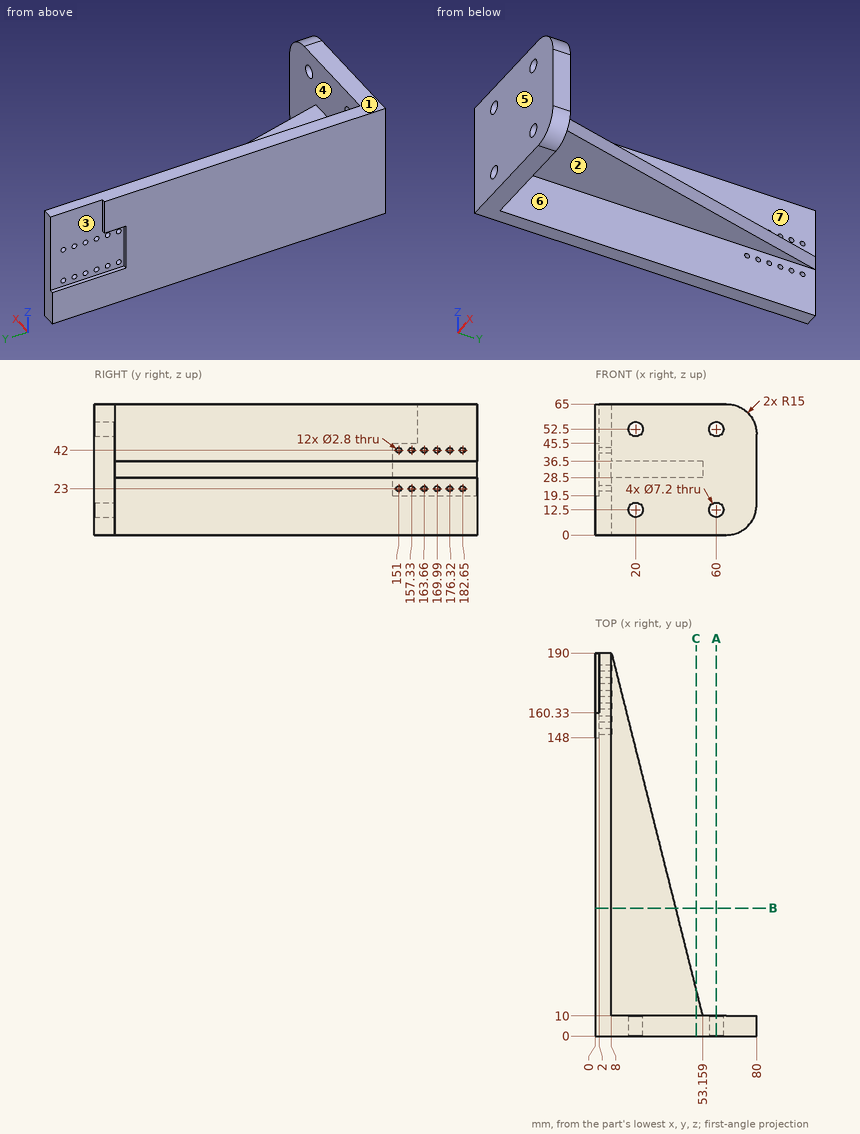
Can you work these out from the drawing? Everything is in mm from the part's minimum corner. A direction names the side the tool comes from. Round coordinates to 2 decimals unless told otherwise and drop trailing zeros. Loops run counter-clockwise (first coordinate to the right, second up) from the corner with the lowest first, then second, coordinate; pieces in that order, holes last. Notation, with made-up numbers: (3, 70) - (39, 70) arc R30 cw to (39, 98) - close; hole circle Ø10 at (85.25, -10.75). An arc over 180 degrees is marked (long way). Answer in a Markdown table with one row per item. Add a question column.
(1) I'm going to push flat-ended pins straight in: pin 1 (6.5 mm diameter, centred on x = 60, z = 52.5, fed in from -Y); pin 2 (12 mm diameter, centred on x = 64.5, z = 44.5, fed in from +Y); pin 3 (3 mm diameter, centred on y = 117, z = 42, fed in from +X); pin 4 (4 mm diameter, centred on x = 17, y = 100.5, fed in from +Z). Where does each tip first touch, or does it pass through?
(2) If we mould it in two halves opening along Z, with no side actions, what happens to the marked faces 1, 2, 3 and 4? For each: pulls with the +Z half, pulls with the -Z half, needs draft (parallel to the pull), parting line crosses it, or undercut.
(3) For the marked faces 5, 6 and 7, which set-ups out of +Z, -Z, +X, -X, +Y, -Y let a thin tool reach every point of the face, with its end or its side?
(4) If we section it at B-B (y = 63.5): Please give me the cut outline in (x, z).
(5) I need wall thicknesses on line 1 along Z through (x, y) = (7, 176); line 2 along X through (y, z) = (3, 52); line 3 along Y through (x, z) = (46, 41). Which ranges of each line are inside material? Lowest first, please.
(6) If we section it at A-A (x = 60): Please give me the cut outline in (y, z), plus the area to 3 significant figures.
(7) If we section it at C-C (x = 50): Please give me the cut outline in (y, z), plus the area to 3 significant figures.
Model answer:
| question | item | result |
|---|---|---|
| 1 | pin 1 | passes through |
| 1 | pin 2 | stops at y = 10 |
| 1 | pin 3 | stops at x = 8 |
| 1 | pin 4 | stops at z = 36.5 |
| 2 | face 1 | pulls with the +Z half |
| 2 | face 2 | pulls with the -Z half |
| 2 | face 3 | undercut |
| 2 | face 4 | needs draft |
| 3 | face 5 | +Z, -Z, +X, -X, -Y |
| 3 | face 6 | -Z, +X, +Y |
| 3 | face 7 | +Z, +X, +Y |
| 4 | outline | (0, 0) - (8, 0) - (8, 28.5) - (39.74, 28.5) - (39.74, 36.5) - (8, 36.5) - (8, 65) - (0, 65) - close |
| 5 | line 1 | z = 0 to 21.64, 24.36 to 40.64, 43.36 to 65 |
| 5 | line 2 | x = 0 to 16.43, 23.57 to 56.43, 63.57 to 79.87 |
| 5 | line 3 | y = 0 to 10 |
| 6 | outline | (0, 0) - (10, 0) - (10, 8.9) - (0, 8.9) - close; (0, 16.1) - (10, 16.1) - (10, 48.9) - (0, 48.9) - close; (0, 56.1) - (10, 56.1) - (10, 65) - (0, 65) - close |
| 6 | area | 506 mm² |
| 7 | outline | (0, 0) - (10, 0) - (10, 28.5) - (22.59, 28.5) - (22.59, 36.5) - (10, 36.5) - (10, 65) - (0, 65) - close |
| 7 | area | 751 mm² |
